```python
from build123d import *

# Parameters (mm, degrees)
SKETCH2_RX              = 31
SKETCH2_RY              = 26
BOSS_EXTRUDE1_DEPTH     = 47
CUT_EXTRUDE1_DEPTH      = 29
CUT_EXTRUDE2_DEPTH      = 27
CUT_EXTRUDE2_DEPTH_BACK = 27
SKETCH5_R               = 4
BOSS_EXTRUDE2_DEPTH     = 17
SKETCH6_W               = 20
SKETCH6_H               = 38.42056209
CUT_EXTRUDE3_DEPTH      = 61.203194114
SKETCH7_R               = 2.5
CUT_EXTRUDE4_DEPTH      = 32.0000001
CUT_EXTRUDE4_DEPTH_BACK = 45.0000001


with BuildPart() as part:
    # Sketch2 → Boss-Extrude1 (new body)
    with BuildSketch(Plane(origin=(0, 0, 0), x_dir=(1, 0, 0), z_dir=(0, 1, 0))):
        with Locations(Location((0, 0), (0, 0, 90))):
            Ellipse(SKETCH2_RX, SKETCH2_RY)
    extrude(amount=BOSS_EXTRUDE1_DEPTH)

    # Sketch3 → Cut-Extrude1 (cut)
    with BuildSketch(Plane.XZ):
        with BuildLine():
            ThreePointArc((-12.714285714, -5.860626142), (14, 0), (-12.714285714, 5.860626142))
            ThreePointArc((-12.714285714, 5.860626142), (-20, 0), (-12.714285714, -5.860626142))
        make_face()
    extrude(amount=-CUT_EXTRUDE1_DEPTH, mode=Mode.SUBTRACT)

    # Sketch4 → Cut-Extrude2 (cut, two sides)
    with BuildSketch(Plane(origin=(0, 0, 0), x_dir=(0, 0, -1), z_dir=(1, 0, 0))) as cut_extrude2_sk:
        Polygon((-3, 47), (31, 38), (31, 47), align=None)
    extrude(amount=CUT_EXTRUDE2_DEPTH, mode=Mode.SUBTRACT)
    extrude(cut_extrude2_sk.sketch, amount=-CUT_EXTRUDE2_DEPTH_BACK, mode=Mode.SUBTRACT)

    # Sketch5 → Boss-Extrude2 (add, symmetric)
    with BuildSketch(Plane(origin=(0, 0, 0), x_dir=(0, 0, -1), z_dir=(1, 0, 0))):
        with BuildLine():
            Line((2.485147451, 45.548049204), (24.5, 58.258330249))
            ThreePointArc((24.5, 58.258330249), (42.258330249, 53.5), (37.5, 35.741669751))
            Line((37.5, 35.741669751), (15.485147451, 23.031388706))
            Line((15.485147451, 23.031388706), (2.485147451, 45.548049204))
        make_face()
        with Locations((31, 47)):
            Circle(SKETCH5_R, mode=Mode.SUBTRACT)
    extrude(amount=BOSS_EXTRUDE2_DEPTH, both=True)

    # Sketch6 → Cut-Extrude3 (cut, through all)
    with BuildSketch(Plane(origin=(0, 33.084936491, 19.101596989), x_dir=(1, 0, 0), z_dir=(0, 0.866025404, 0.5))):
        with Locations((0, 44.136506472)):
            Rectangle(SKETCH6_W, SKETCH6_H)
    extrude(amount=-CUT_EXTRUDE3_DEPTH, mode=Mode.SUBTRACT)

    # Sketch7 → Cut-Extrude4 (cut, two sides)
    with BuildSketch(Plane.XY) as cut_extrude4_sk:
        with Locations((20, 29.844780472)):
            Circle(SKETCH7_R)
        with Locations((20, 17.844780472)):
            Circle(SKETCH7_R)
    extrude(amount=CUT_EXTRUDE4_DEPTH, mode=Mode.SUBTRACT)
    extrude(cut_extrude4_sk.sketch, amount=-CUT_EXTRUDE4_DEPTH_BACK, mode=Mode.SUBTRACT)


solid = part.part
```
The model under review builds one solid part; all positions refer to its coordinate system, in mm. A direction names the side the tool comes from. Round coordinates to 2 decimals unless told otherwise and drop trailing zeros. Write each loop counter-clockwise with the first axis right and the second up, starting at its lowest first coordinate (ties: lowest second). Pieces come first, ordered by that corner, then holes. Notation, with made-up numbers: (36, -20) - (42, -20) arc R26 ccw to (42, -6) - close; hole circle Ø6 at (7.5, 14.5). An arc over 180 degrees is marked (long way). Answer as CSV lines item,"result". Start each with the question number.
(1) We need section A-A on z = -31. State the section outline as (x, y) points, plus the area to 3 significant figures.
(2) Draft analysis for pull direction X (two halves, no side actions). For faces 4 (the cylindrical face through (13.99, 14.3, -0.53)), 5 (the flat face through (13.549, 51.814, -13.338)), 6 (the flat face through (-17, 44, -28)), state which applies: pulls with the +X half, pulls with the -X half, needs draft (parallel to the pull), parting line crosses it, or undercut.
(3) For faces 1 (the flat face through (-13.451, 32.645, -32.137)), 2 (the flat face through (13.549, 32.645, -32.137)), 3 (the cylindrical face through (-20, 14, 0)), list the 3-axis set-ups (+Z, -Z, +X, -X, +Y, -Y) from which the entire face can be reached by the end or side of a thin tool; tool diameter is ignored.
(4) We need section B-B on x = 20. Give the number of separate pieces and of enclosed holes in the cut face, plus the area to 3 significant figures.
(5) For pin 1 Ø5 at (x, y) = (8, 25) entering from -Z; pin 2 Ø2 at (x, y) = (1, 41) entering from +Z; pin 3 Ø12.5 at (y, z) = (16.5, -30.5) entering from +X; pin 4 Ø5 at (x, z) = (-0.5, -17.5) entering from -Y, all flat-tipped, find the tip position at first contact; note any pin that passes through.
(6) To check wall thickness, follow line 1 (Y direction, x = 20, z = -16.25); line 2 (Y direction, x = 20, z = -16.5); line 3 (Y direction, x = 16.5, z = 21.5). State the ranges of each line that lie inside material, in increasing order.
Worked answers:
1,outline,"(-17, 31.99) - (-10, 31.99) - (-10, 43) - (-17, 43) - close; (-17, 51) - (-10, 51) - (-10, 60) - (-17, 60) - close; (10, 31.99) - (17, 31.99) - (17, 43) - (10, 43) - close; (10, 51) - (17, 51) - (17, 60) - (10, 60) - close"
1,area,"280 mm²"
2,face 4,"undercut"
2,face 5,"needs draft"
2,face 6,"pulls with the -X half"
3,face 1,"-Z, -X, -Y"
3,face 2,"-Z, +X, -Y"
3,face 3,"-Y"
4,separate pieces,"3"
4,enclosed holes,"0"
4,area,"1,400 mm²"
5,pin 1,"z = -28.62"
5,pin 2,"z = 31"
5,pin 3,"x = 16.2"
5,pin 4,"y = 0"
6,line 1,"0 to 15.34, 20.34 to 27.34, 32.34 to 41.9"
6,line 2,"0 to 15.34, 20.34 to 27.34, 32.34 to 41.84"
6,line 3,"0 to 47"
